The listing builds one solid part. Answer for the finished solid, in the listing's coordinates (mm). A direction names the side the tool comes from. Round coordinates to 2 decimals unless told otherwise and drop trailing zeros. Write each loop counter-clockwise with the first axis right and the second up, starting at its lowest first coordinate (ties: lowest second). Pieces come first, ordered by that corner, then holes. Notation, with made-up numbers: (48, 63) - (83, 63) arc R22 cw to (83, 102) - close; hole circle Ø9 at (78, 25.25). An arc over 180 degrees is marked (long way). Answer as CSV lines item,"result". Start each with the question number.
Item 1: A cutting plane is placed at C-C on z = 8.5. Determine the outline of the cut face in (x, y), and give its area (3 significant figures).
Item 2: A cutting plane is placed at D-D on z = 25.5. Determine the outline of the cut face in (x, y), and give its area (3 significant figures).
Item 3: Straight lines are drawn through the part: line 1 along Y through (x, z) = (0, 8.5); line 2 along X through (y, z) = (0, 14.5); line 3 along Y through (x, z) = (9.5, 21). For each, find the intervals that lie inside material, in ascending order. Write a range as [from, to].
Item 4: Which of the six approach directions +Z, -Z, +X, -X, +Y, -Y give full straight-line access (tool end or side, diameter ignored) to faces 1 (the cylindrical face through (0, 45, 7)), 2 (the flat face through (0, 22, 21)), 3 (the flat face through (7, 21, 0))?
Item 5: Flat-ended cylindrical pins translate along their axes: pin 1 (3 mm diameter, centred on y = -5.5, z = 4, fed in from -X); pin 2 (3.5 mm diameter, centred on y = 20.5, z = 29.5, fed in from -X); pin 3 (1.5 mm diameter, centred on y = -10.5, z = 34.5, fed in from +X). Find the tip coordinate at first contact, or state that the pin passes through.
Item 6: A cutting plane is placed at B-B on x = 11. Determine the outline of the cut face in (y, z), and give its area (3 significant figures).
Item 7: A cutting plane is placed at A-A on y = 4.5. Determine the outline of the cut face in (x, z).
Item 8: For a pull along X with two mould halves and no side action, classify faces 4 (the flat face through (-4.5, 20, 21)), 5 (the flat face through (7, 21, 42)), 6 (the cylindrical face through (28.568, -9.905, 21.294)) as pulls with the +X half, pulls with the -X half, needs draft (parallel to the pull), parting line crosses it, or undercut.
```python
from build123d import *

# Parameters (mm, degrees)
ESQUISSE1_W                        = 36
ESQUISSE1_H                        = 42
ENL_V_MAT_EXTRU_1_REACH            = 75.239
ESQUISSE3_W                        = 18
ESQUISSE3_H                        = 42
DIAM_TRE_DU_PER_AGE_M6_0_6_1_D     = 6
DIAM_TRE_DU_PER_AGE_M6_0_6_1_DEPTH = 14
DIAM_TRE_DU_PER_AGE_M6_0_6_1_TIP   = 1.732050808


with BuildPart() as part:
    # Esquisse1 → Révolution1 (revolve)
    with BuildSketch(Plane.XZ.offset(-12), mode=Mode.PRIVATE) as r_volution1_sk:
        with Locations((18, 21)):
            Rectangle(ESQUISSE1_W, ESQUISSE1_H)
    revolve(r_volution1_sk.sketch.rotate(Axis((0, 12, 42), (0, 0, -1)), 180), axis=Axis((0, 12, 42), (0, 0, -1)))

    # Esquisse2 → Enlèv. mat.-Extru.1 (cut, up to next)
    with BuildSketch(Plane(origin=(0, 0, 0), x_dir=(-1, 0, 0), z_dir=(0, 0, -1)), mode=Mode.PRIVATE) as enl_v_mat_extru_1_sk1:
        with BuildLine():
            Line((4.5, 22), (-4.5, 22))
            Line((-4.5, 22), (-4.5, 17.428425058))
            ThreePointArc((-4.5, 17.428425058), (0, 18), (4.5, 17.428425058))
            Line((4.5, 17.428425058), (4.5, 22))
        make_face()
    enl_v_mat_extru_1_tool1 = extrude(enl_v_mat_extru_1_sk1.sketch, amount=-ENL_V_MAT_EXTRU_1_REACH, mode=Mode.PRIVATE) & part.part
    add(enl_v_mat_extru_1_tool1.solids().sort_by_distance((0, 19.901901, 0))[0], mode=Mode.SUBTRACT)

    # Esquisse3 → Enlèvement de matière-Révolution1 (revolve, cut)
    with BuildSketch(Plane(origin=(0, 0, 0), x_dir=(1, 0, 0), z_dir=(0, 1, 0))):
        with Locations((9, -21)):
            Rectangle(ESQUISSE3_W, ESQUISSE3_H)
    revolve(axis=Axis((0, 0, 0), (0, 0, 1)), mode=Mode.SUBTRACT)

    # Diamètre du perçage M6.0 (6)1
    with Locations(Plane(origin=(0, 0, 0), x_dir=(-1, 0, 0), z_dir=(0, 0, -1))):
        with Locations((0, 42)):
            Hole(DIAM_TRE_DU_PER_AGE_M6_0_6_1_D / 2, depth=DIAM_TRE_DU_PER_AGE_M6_0_6_1_DEPTH)
            with Locations((0, 0, -(DIAM_TRE_DU_PER_AGE_M6_0_6_1_DEPTH + DIAM_TRE_DU_PER_AGE_M6_0_6_1_TIP / 2))):  # 120° drill point
                Cone(0, DIAM_TRE_DU_PER_AGE_M6_0_6_1_D / 2, DIAM_TRE_DU_PER_AGE_M6_0_6_1_TIP, mode=Mode.SUBTRACT)


solid = part.part
```
Geometry says:
1,outline,"circle Ø72 at (0, 12); hole (-4.5, 17.43) arc R18 ccw (long way) to (4.5, 17.43) - (4.5, 22) - (-4.5, 22) - close; hole circle Ø6 at (0, 42)"
1,area,"2,990 mm^2"
2,outline,"circle Ø72 at (0, 12); hole (-4.5, 17.43) arc R18 ccw (long way) to (4.5, 17.43) - (4.5, 22) - (-4.5, 22) - close"
2,area,"3,020 mm^2"
3,line 1,"y = [-24, -18], [22, 39], [45, 48]"
3,line 2,"x = [-33.94, -18], [18, 33.94]"
3,line 3,"y = [-22.72, -15.29], [15.29, 46.72]"
4,face 1,"-Z"
4,face 2,"+Z, -Z"
4,face 3,"-Z, +X, -X, +Y, -Y"
5,pin 1,"stops at x = -32.25"
5,pin 2,"stops at x = -35.36"
5,pin 3,"stops at x = 28.69"
6,outline,"(-22.28, 0) - (-14.25, 0) - (-14.25, 42) - (-22.28, 42) - close; (14.25, 0) - (46.28, 0) - (46.28, 42) - (14.25, 42) - close"
6,area,"1,680 mm^2"
7,outline,"(-35.21, 0) - (-17.43, 0) - (-17.43, 42) - (-35.21, 42) - close; (17.43, 0) - (35.21, 0) - (35.21, 42) - (17.43, 42) - close"
8,face 4,"undercut"
8,face 5,"needs draft"
8,face 6,"parting line crosses it"
